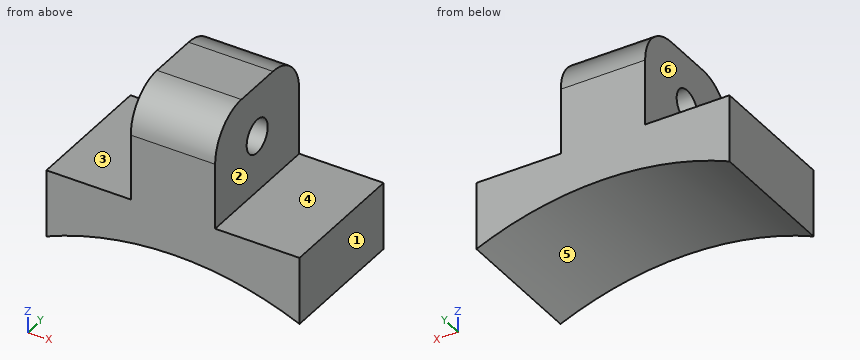
from build123d import *

# Parameters (mm, degrees)
EXTRUDE_START       = 6
EXTRUDE_1_DEPTH     = 16
EXTRUDE_2_DEPTH     = 5
SKETCH_3_R          = 2
CUT_EXTRUDE_1_DEPTH = 15


with BuildPart() as part:
    # Эскиз1 → Вытянуть1 (new body)
    with BuildSketch(Plane(origin=(0, 0, 0), x_dir=(1, 0, 0), z_dir=(0, 1, 0)).offset(EXTRUDE_START)):
        with BuildLine():
            Line((-15, -34.9141805), (-15, -42.9141805))
            Line((-15, -42.9141805), (15, -42.9141805))
            Line((15, -42.9141805), (15, -34.9141805))
            ThreePointArc((15, -34.9141805), (0, -38), (-15, -34.9141805))
        make_face()
    extrude(amount=EXTRUDE_1_DEPTH)

    # Эскиз2 → Вытянуть2 (add, symmetric)
    with BuildSketch(Plane(origin=(0, 0, 0), x_dir=(0, 0, -1), z_dir=(1, 0, 0))):
        with BuildLine():
            Line((-42.9141805, 22), (-50.712858665, 22))
            ThreePointArc((-50.712858665, 22), (-54.248392571, 20.535533906), (-55.712858665, 17))
            Line((-55.712858665, 17), (-55.712858665, 11))
            ThreePointArc((-55.712858665, 11), (-54.248392571, 7.464466094), (-50.712858665, 6))
            Line((-50.712858665, 6), (-42.9141805, 6))
            Line((-42.9141805, 6), (-42.9141805, 22))
        make_face()
    extrude(amount=EXTRUDE_2_DEPTH, both=True)

    # Эскиз3 → Вырез-Вытянуть1 (cut, symmetric)
    with BuildSketch(Plane.ZY.offset(5)):
        with Locations((49.571306652, 14)):
            Circle(SKETCH_3_R)
    extrude(amount=CUT_EXTRUDE_1_DEPTH, both=True, mode=Mode.SUBTRACT)


solid = part.part
Model file for the job. Use its own axes, mm. Face numbers are marked on the shaded views. A direction names the side the tool comes from. Give positions to 0.01 mm unless a question says otherwise; leave off trailing zeros. Loops run counter-clockwise (first coordinate to the right, second up) from the corner with the lowest first, then second, coordinate; pieces in that order, holes last. Notation, with made-up numbers: (-9, 50) -> (10, 50) arc R23 ccw to (10, 62) -> close; hole circle Ø8 at (22.5, -3.75). An arc over 180 degrees is marked (long way). Use a Markdown table: item, result. Add a question column.
(1) Slice it at B-B on z = 50. List the corners of the cut face in (x, y), and give its area (3 significant figures).
(2) Mould opens along X. For the marked faces 4, 5 and 6 say: +X half, -X half, draft (parallel to the pull), parting line (faces both ways), or undercut.
(3) Wall check: line 1 along X through (y, z) = (13.75, 54.25); line 2 along Z through (x, y) = (-6.25, 17); line 3 along Z through (x, y) = (9, 10.5). Give the ranges that are in metal, low to high.
(4) Drop flat-ended pins along their axis: pin 1 Ø3 at (x, y) = (10, 15) entering from +Z; pin 2 Ø4.5 at (y, z) = (14, 49.57) entering from +X; pin 3 Ø2 at (y, z) = (20, 47) entering from -X. Give the stop position or say it passes through.
(5) Slice it at A-A on y = 14. List the corners of the cut face in (x, z).
(6) Slice it at D-D on y = 18. List the corners of the cut face in (x, z), and give its area (3 significant figures).
(7) Slice it at C-C on x = -0.75. List the corners of the cut face in (y, z), and give its area (3 significant figures).
(8) Tool access for the marked faces 1, 2 and 3: list every direction of +Z, -Z, +X, -X, +Y, -Y with a clear straight run to the whole face (end or side of a thin tool).
Filled sheet:
| question | item | result |
|---|---|---|
| 1 | outline | (-5, 6) -> (5, 6) -> (5, 12.05) -> (-5, 12.05) -> close; (-5, 15.95) -> (5, 15.95) -> (5, 22) -> (-5, 22) -> close |
| 1 | area | 121 mm2 |
| 2 | face 4 | draft |
| 2 | face 5 | undercut |
| 2 | face 6 | -X half |
| 3 | line 1 | -5 to 5 |
| 3 | line 2 | 37.48 to 42.91 |
| 3 | line 3 | 36.92 to 42.91 |
| 4 | pin 1 | z = 42.91 |
| 4 | pin 2 | x = 5 |
| 4 | pin 3 | x = -5 |
| 5 | outline | (-15, 34.91) arc R38 cw to (15, 34.91) -> (15, 42.91) -> (5, 42.91) -> (5, 47.57) -> (-5, 47.57) -> (-5, 42.91) -> (-15, 42.91) -> close; (-5, 51.57) -> (5, 51.57) -> (5, 55.71) -> (-5, 55.71) -> close |
| 6 | outline | (-15, 34.91) arc R38 cw to (15, 34.91) -> (15, 42.91) -> (5, 42.91) -> (5, 55.61) -> (-5, 55.61) -> (-5, 42.91) -> (-15, 42.91) -> close |
| 6 | area | 305 mm2 |
| 7 | outline | (6, 37.99) -> (22, 37.99) -> (22, 50.71) arc R5 ccw to (17, 55.71) -> (11, 55.71) arc R5 ccw to (6, 50.71) -> close; hole circle Ø4 at (14, 49.57) |
| 7 | area | 260 mm2 |
| 8 | face 1 | +Z, -Z, +X, +Y, -Y |
| 8 | face 2 | +Z, +X, +Y, -Y |
| 8 | face 3 | +Z, -X, +Y, -Y |
